Could you check a few things on this model? Use its own coordinates, in mm. Round coordinates to 2 decimals unless told otherwise and drop trailing zeros. Loops run counter-clockwise (first coordinate to the right, second up) from the corner with the lowest first, then second, coordinate; pieces in that order, holes last. Notation, with made-up numbers: (29.25, 32.25) -> (54.25, 32.25) arc R11 cw to (54.25, 45.25) -> close; hole circle Ø3 at (7.25, 1.5). An arc over 180 degrees is marked (long way). One line per item, written item: value.
```python
from build123d import *

# Parameters (mm, degrees)
SKETCH1_R           = 65
SKETCH1_R_2         = 40
SKETCH1_R_3         = 3.05
BOSS_EXTRUDE1_DEPTH = 15
SKETCH2_R           = 3
CUT_EXTRUDE1_DEPTH  = 94.139680051
CIRPATTERN1_COUNT   = 6


with BuildPart() as part:
    # Sketch1 → Boss-Extrude1 (new body)
    with BuildSketch(Plane(origin=(0, 0, 0), x_dir=(1, 0, 0), z_dir=(0, 1, 0))):
        with Locations(Location((0, 0, 0), (0, 0, 270))):
            Circle(SKETCH1_R)
        with Locations(Location((0, 0, 0), (0, 0, 270))):
            Circle(SKETCH1_R_2, mode=Mode.SUBTRACT)
        with Locations(Location((12.723046489, -48.354152749, 0), (0, 0, 270))):
            Circle(SKETCH1_R_3, mode=Mode.SUBTRACT)
    extrude(amount=BOSS_EXTRUDE1_DEPTH)

    # Sketch2 → Cut-Extrude1 (cut, through all)
    with BuildSketch(Plane(origin=(0, 0, 0), x_dir=(0, 0, -1), z_dir=(1, 0, 0))):
        with Locations((0, 7.5)):
            Circle(SKETCH2_R)
    cut_extrude1 = extrude(amount=-CUT_EXTRUDE1_DEPTH, mode=Mode.SUBTRACT)

    # CirPattern1: Cut-Extrude1 ×6 about axis
    cirpattern1_axis = Axis((0, 15, 0), (0, 1, 0))
    for i in range(1, CIRPATTERN1_COUNT):
        add(cut_extrude1.rotate(cirpattern1_axis, i * 360 / CIRPATTERN1_COUNT), mode=Mode.SUBTRACT)


solid = part.part
```
(1) Imagine slicing it at A-A on x = 0. Write out the boundary of the cut face in (y, z), then the cut area to 3 significant figures.
Results below:
outline: (0, -65) -> (15, -65) -> (15, -40) -> (0, -40) -> close; (0, 40) -> (15, 40) -> (15, 65) -> (0, 65) -> close
area: 750 mm²
(2) Imagine slicing it at D-D on x = -14. Write out the boundary of the cut face in (y, z), then the cut area to 3 significant figures.
Results below:
outline: (0, -63.47) -> (15, -63.47) -> (15, -37.47) -> (0, -37.47) -> close; (0, 37.47) -> (15, 37.47) -> (15, 63.47) -> (0, 63.47) -> close
area: 780 mm²
(3) Imagine slicing it at C-C on x = 44. Write out the boundary of the cut face in (y, z).
Results below:
outline: (0, -47.84) -> (15, -47.84) -> (15, 47.84) -> (0, 47.84) -> close; hole circle Ø6 at (7.5, 0)
(4) Please list where these lines run through material, in increasing order: L1, parallel to X at y = 11.5, z = 0; L2, parallel to Z at x = -28, y = 9.5; L3, parallel to X at y = 8.75, z = -42.
Results below:
L1: x = -65 to -40, 40 to 65
L2: z = -58.66 to -52.97, -44.03 to -28.57, 28.57 to 44.03, 52.97 to 58.66
L3: x = -49.61 to -27.4, -21.1 to 21.1, 27.4 to 49.61
(5) For pin 1 Ø1.5 at (x, y) = (-17, 11) entering from -Z; pin 2 Ø5 at (y, z) = (11, 3) entering from +X; pin 3 Ø4 at (y, z) = (9.5, 21) entering from -X, each with a flat end and sliding along its axis, tell me the tip position at first contact or that it passes through.
Results below:
pin 1: stops at z = -62.94
pin 2: stops at x = 65
pin 3: stops at x = -62.16
(6) Imagine slicing it at B-B on y = 9. Write out the boundary of the cut face in (x, z), then the cut area to 3 significant figures.
Results below:
outline: (-64.95, -2.6) arc R65 ccw to (-34.72, -54.95) -> (-22.21, -33.27) arc R40 cw to (-39.92, -2.6) -> close; (-64.95, 2.6) -> (-39.92, 2.6) arc R40 cw to (-22.21, 33.27) -> (-34.72, 54.95) arc R65 ccw to start; (-30.22, -57.55) arc R65 ccw to (30.22, -57.55) -> (17.71, -35.87) arc R40 cw to (-17.71, -35.87) -> close; (-30.22, 57.55) -> (-17.71, 35.87) arc R40 cw to (17.71, 35.87) -> (30.22, 57.55) arc R65 ccw to start; (22.21, -33.27) -> (34.72, -54.95) arc R65 ccw to (64.95, -2.6) -> (39.92, -2.6) arc R40 cw to start; (22.21, 33.27) arc R40 cw to (39.92, 2.6) -> (64.95, 2.6) arc R65 ccw to (34.72, 54.95) -> close; hole circle Ø6.1 at (12.72, 48.35)
area: 7,440 mm²
(7) We'd pull the mould along Z, two halves only. Please class faces 1 (the face through (-23.66, 8.4, -46.7)), 2 (the face through (30, 0, 28)), 3 (the face through (19.52, 7.4, 62)): +Z half, -Z half, draft (parallel to the pull), parting line (faces both ways), or undercut.
Results below:
face 1: undercut
face 2: draft
face 3: parting line
